For this review, take the finished solid that the model builds, in its own axes (mm). Face numbers are marked on the shaded views. Give positions to 0.01 mm unless a question says otherwise; leave off trailing zeros. Order: outer loops, then holes, each group sorted by start corner. A loop starts at its lowest first (then second) coordinate and runs counter-clockwise, first axis right, second up.
from build123d import *

# Parameters (mm, degrees)
F0_R     = 6.5
F1_DEPTH = 15
F2_R     = 3
F2_R_2   = 1.5
F3_DEPTH = 5
F4_R     = 3.49999
F5_R     = 3


# Not quite as in the source:
# - a fillet or chamfer is up to 0.001 mm smaller than in the source, because OpenCascade refuses the exact size


with BuildPart() as f1:
    # F0 (on Top) → F1 (new body)
    with BuildSketch(Plane.XY):
        Circle(F0_R)
    extrude(amount=F1_DEPTH)

    # F2 (on face) → F3 (join)
    with BuildSketch(Plane(origin=(0, 0, 0), x_dir=(1, 0, 0), z_dir=(0, 0, -1))):
        Circle(F2_R)
        Circle(F2_R_2, mode=Mode.SUBTRACT)
    extrude(amount=F3_DEPTH)

    # F4 (radius 3.5 in the source; OpenCascade refuses exactly that, so slightly less here)
    f4_edges = [f1.edges().sort_by_distance(p)[0] for p in [
        (-6.5, 0, 0),
    ]]
    fillet(f4_edges, radius=F4_R)

    # F5
    f5_edges = [f1.edges().sort_by_distance(p)[0] for p in [
        (-6.5, 0, 15),
    ]]
    fillet(f5_edges, radius=F5_R)


solid = f1.part
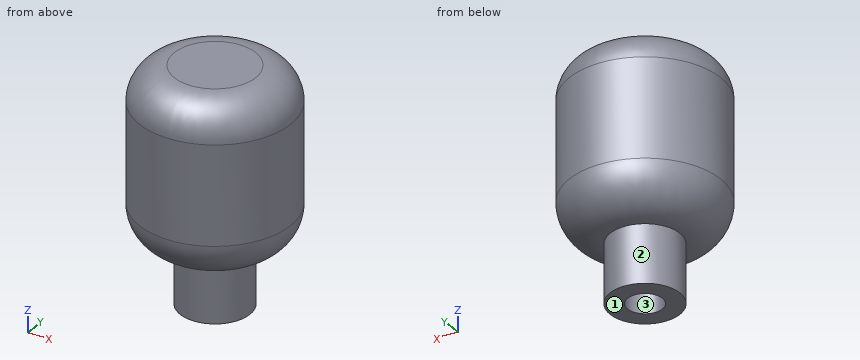
1) Clearance check with flat-ended pins moving along their axes: pin 1 (1.5 mm diameter, centred on x = 0.5, y = 0, fed in from -Z); pin 2 (1 mm diameter, centred on x = 4, y = -1.5, fed in from -Z); pin 3 (1 mm diameter, centred on x = 5, y = 0, fed in from +Z). State where each tip first meets the part, or that it passes through.
Answer sheet:
pin 1: stops at z = 0
pin 2: stops at z = 0.09
pin 3: stops at z = 14.83
2) To check wall thickness, follow line 1 (X direction, y = 0, z = -3.85); line 2 (X direction, y = -2, z = 8.25). State the ranges of each line that lie inside material, in increasing order.
Answer sheet:
line 1: x = -3 to -1.5, 1.5 to 3
line 2: x = -6.18 to 6.18
3) Draft analysis for pull direction X (two halves, no side actions). For the marked faces 1, 2 and 3, state which applies: +X half, -X half, draft (parallel to the pull), parting line (faces both ways), or undercut.
Answer sheet:
face 1: draft
face 2: parting line
face 3: undercut
4) We need section A-A on z = 4.5. Give the boundary of the cut face in (x, y).
Answer sheet:
outline: circle Ø13 at (0, 0)
